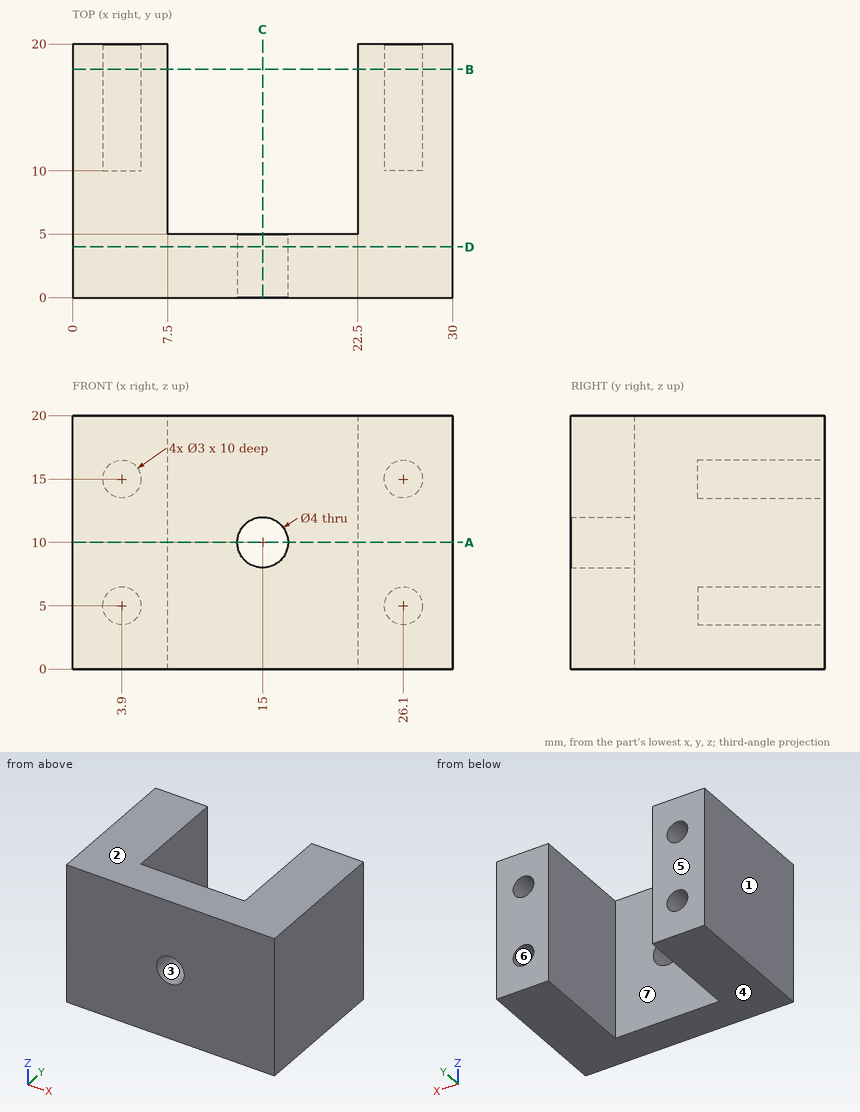
Input: dimensioned drawing with shaded views. Units: mm. Origin: part minimum x, y, z. A direction names the side the tool comes from. Coordinates: 2 decimals unless noted, no trailing zeros. Write each loop counter-clockwise with the first axis right and the second up, starting at its lowest first coordinate (ties: lowest second). Pieces come first, ordered by that corner, then holes. Notation, with made-up numbers: (71.25, -7) -> (91.25, -7) arc R25 ccw to (91.25, 32) -> close; hole circle Ø10 at (-11, 16.25). An arc over 180 degrees is marked (long way). Return JSON: item names as keys, results as strings. Group by question number.
1) Mould query, pull axis Z, two halves, no side actions, for the marked faces 1, 2, 3 and 4. Classes: +Z half, -Z half, draft (parallel to the pull), parting line (faces both ways), or undercut.
2) Section query A-A, the plane z = 10. Return loops of the section in (x, y).
3) Section query C-C, the plane x = 15. Return loops of the section in (y, z), plus the area to 3 significant figures.
4) Contact query for flat-ended pins moving along their axis: P1, Ø7.5, axis at x = 17.5, z = 14.5, coming from the +Y side; P2, Ø2.5, axis at x = 26.1, z = 5, coming from the +Y side. Output: stop coordinate, or through.
5) Section query D-D, the plane y = 4. Return loops of the section in (x, z).
6) Section query B-B, the plane y = 18. Return loops of the section in (x, z), plus the area to 3 significant figures.
7) Ray query, line 1 along Z through (x, y) = (3.9, 12.5); line 2 along X through (y, z) = (16, 1.75); line 3 along Z through (x, y) = (15, 1.1). Return the intervals inside material, ascending.
8) Set-up query: the marked faces 5, 6 and 7. Return all of +Z, -Z, +X, -X, +Y, -Y with unobstructed straight access to the full face (end or side cutting, diameter ignored); none if empty.
From the geometry:
{
 "1": {"face 1": "draft", "face 2": "+Z half", "face 3": "undercut", "face 4": "-Z half"},
 "2": {"outline": "(0, 0) -> (13, 0) -> (13, 5) -> (7.5, 5) -> (7.5, 20) -> (0, 20) -> close; (17, 0) -> (30, 0) -> (30, 20) -> (22.5, 20) -> (22.5, 5) -> (17, 5) -> close"},
 "3": {"outline": "(0, 0) -> (5, 0) -> (5, 8) -> (0, 8) -> close; (0, 12) -> (5, 12) -> (5, 20) -> (0, 20) -> close", "area": "80.0 mm²"},
 "4": {"P1": "y = 5", "P2": "y = 10"},
 "5": {"outline": "(0, 0) -> (30, 0) -> (30, 20) -> (0, 20) -> close; hole circle Ø4 at (15, 10)"},
 "6": {"outline": "(0, 0) -> (7.5, 0) -> (7.5, 20) -> (0, 20) -> close; (22.5, 0) -> (30, 0) -> (30, 20) -> (22.5, 20) -> close; hole circle Ø3 at (3.9, 5); hole circle Ø3 at (3.9, 15); hole circle Ø3 at (26.1, 5); hole circle Ø3 at (26.1, 15)", "area": "272 mm²"},
 "7": {"line 1": "0 to 3.5, 6.5 to 13.5, 16.5 to 20", "line 2": "0 to 7.5, 22.5 to 30", "line 3": "0 to 8, 12 to 20"},
 "8": {"face 5": "+Z, -Z, +X, -X, +Y", "face 6": "+Y", "face 7": "+Z, -Z, +Y"}
}
